Build history of the part. All positions in model axes, mm. Face numbers are marked on the shaded views. A direction names the side the tool comes from. Coordinates: 2 decimals unless noted, no trailing zeros. Loops run counter-clockwise (first coordinate to the right, second up) from the corner with the lowest first, then second, coordinate; pieces in that order, holes last.
Item 1: Cut at A-A (z = 0). List the corners of the cut face in (x, y), and give its area (3 significant figures).
Item 2: Cut at C-C (x = 6). List the corners of the cut face in (y, z), and give its area (3 significant figures).
Item 3: Mould opens along Y. For the marked faces 1, 2, 3 and 4 say: released by +Y, released by -Y, zero draft, split by the parting line, or undercut.
Item 4: Cut at B-B (y = 0). List the corners of the cut face in (x, z), and give its area (3 significant figures).
Item 5: Drill centre lines: line 1 along Y through (x, z) = (4.25, 0); line 2 along Z through (x, y) = (10.75, -0.5); line 3 along Y through (x, z) = (0.85, 0). Where is each one in solid material? Low to high.
Item 6: Cut at D-D (z = -19). List the corners of the cut face in (x, y).
Item 7: Flat gauge pins, fed straight in: pin 1 (25 mm diameter, centred on y = -10, z = 4.5, fed in from +X); pin 2 (1.2 mm diameter, centred on x = 11.5, z = -24, fed in from -Y); pin 3 (0.6 mm diameter, centred on x = 10.5, y = -2, fed in from +Z). Where does each tip first touch, or does it go through?
Item 8: 3-axis set-ups, long thin cutter, end or side, ignore diameter. For the marked faces 5, 6 and 7: which of +Z, -Z, +X, -X, +Y, -Y reach the whole face in a straight line?
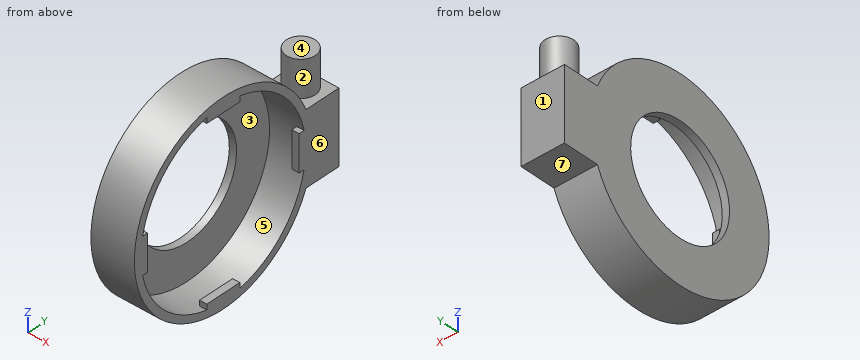
from build123d import *

# Parameters (mm, degrees)
SKETCH1_R           = 15
BOSS_EXTRUDE1_DEPTH = 12
SKETCH2_R           = 25
CUT_EXTRUDE1_DEPTH  = 10
SKETCH3_R           = 4
BOSS_EXTRUDE2_DEPTH = 10
BOSS_EXTRUDE3_DEPTH = 2


with BuildPart() as part:
    # Sketch1 → Boss-Extrude1 (new body)
    with BuildSketch(Plane(origin=(0, 0, 0), x_dir=(0, 0, -1), z_dir=(1, 0, 0))):
        with BuildLine():
            Line((-10, 25.079872408), (-10, 35.079872408))
            Line((-10, 35.079872408), (10, 35.079872408))
            Line((10, 35.079872408), (10, 25.079872408))
            ThreePointArc((10, 25.079872408), (0, -27), (-10, 25.079872408))
        make_face()
        Circle(SKETCH1_R, mode=Mode.SUBTRACT)
    extrude(amount=BOSS_EXTRUDE1_DEPTH)

    # Sketch2 → Cut-Extrude1 (cut)
    with BuildSketch(Plane(origin=(12, 0, 0), x_dir=(0, 0, -1), z_dir=(1, 0, 0))):
        Circle(SKETCH2_R)
    extrude(amount=-CUT_EXTRUDE1_DEPTH, mode=Mode.SUBTRACT)

    # Sketch3 → Boss-Extrude2 (add)
    with BuildSketch(Plane.XY.offset(10)):
        with Locations(Location((6, 30.079872408, 0), (0, 0, 180))):
            Circle(SKETCH3_R)
    extrude(amount=BOSS_EXTRUDE2_DEPTH)

    # Sketch4 → Boss-Extrude3 (add)
    with BuildSketch(Plane(origin=(12, 0, 0), x_dir=(0, 0, -1), z_dir=(1, 0, 0))):
        with BuildLine():
            Line((-23, 5), (-24.494897428, 5))
            ThreePointArc((-24.494897428, 5), (-25, 0), (-24.494897428, -5))
            Line((-24.494897428, -5), (-23, -5))
            Line((-23, -5), (-23, 5))
        make_face()
        with BuildLine():
            ThreePointArc((5, 24.494897428), (0, 25), (-5, 24.494897428))
            Line((-5, 24.494897428), (-5, 23))
            Line((-5, 23), (5, 23))
            Line((5, 23), (5, 24.494897428))
        make_face()
        with BuildLine():
            ThreePointArc((25, 0), (24.873403825, 2.51272405), (24.494897428, 5))
            Line((24.494897428, 5), (23, 5))
            Line((23, 5), (23, -5))
            Line((23, -5), (24.494897428, -5))
            ThreePointArc((24.494897428, -5), (24.873403825, -2.51272405), (25, 0))
        make_face()
        with BuildLine():
            Line((-5, -23), (-5, -24.494897428))
            ThreePointArc((-5, -24.494897428), (0, -25), (5, -24.494897428))
            Line((5, -24.494897428), (5, -23))
            Line((5, -23), (-5, -23))
        make_face()
    extrude(amount=-BOSS_EXTRUDE3_DEPTH)


solid = part.part
Filled sheet:
1. outline: (0, -27) - (12, -27) - (12, -23) - (10, -23) - (10, -25) - (2, -25) - (2, -15) - (0, -15) - close; (0, 15) - (2, 15) - (2, 25) - (10, 25) - (10, 23) - (12, 23) - (12, 35.08) - (0, 35.08) - close
1. area: 193 mm2
2. outline: (25.08, -10) - (35.08, -10) - (35.08, 10) - (34.08, 10) - (34.08, 20) - (26.08, 20) - (26.08, 10) - (25.08, 10) arc R27 ccw (long way) to start; hole circle Ø50 at (0, 0)
2. area: 581 mm2
3. face 1: released by +Y
3. face 2: undercut
3. face 3: undercut
3. face 4: zero draft
4. outline: (0, -27) - (12, -27) - (12, -23) - (10, -23) - (10, -25) - (2, -25) - (2, -15) - (0, -15) - close; (0, 15) - (2, 15) - (2, 25) - (10, 25) - (10, 23) - (12, 23) - (12, 27) - (0, 27) - close
4. area: 96.0 mm2
5. line 1: y = -27 to -25, 25 to 35.08
5. line 2: z = -27 to -23, 23 to 27
5. line 3: y = -27 to -15, 15 to 35.08
6. outline: (0, -19.18) - (12, -19.18) - (12, -16.25) - (2, -16.25) - (2, 16.25) - (12, 16.25) - (12, 19.18) - (0, 19.18) - close
7. pin 1: stops at x = 2
7. pin 2: stops at y = -13.47
7. pin 3: stops at z = 26.95
8. face 5: none
8. face 6: +Z, -Z, +X, +Y, -Y
8. face 7: -Z, +X, -X, +Y
